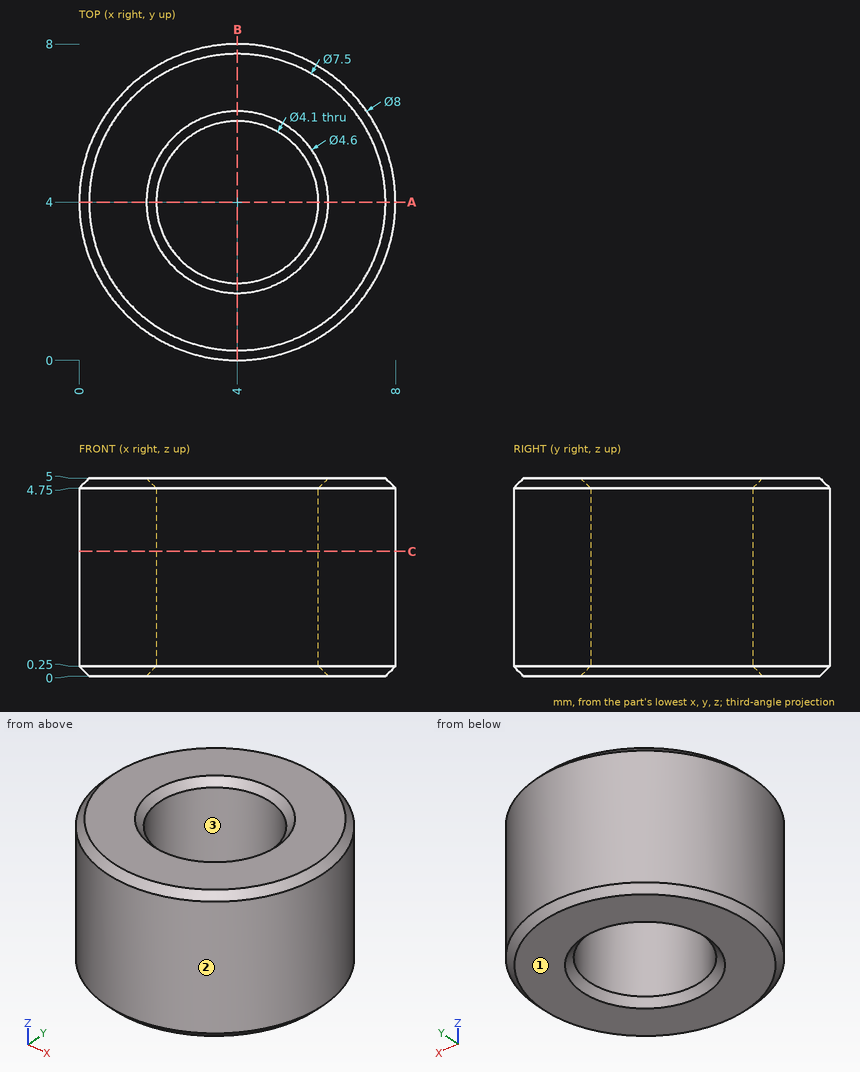
Can you work these out from the drawing? Everything is in mm from the part's minimum corner. Round coordinates to 2 decimals unless told otherwise and drop trailing zeros. Loops run counter-clockwise (first coordinate to the right, second up) from the corner with the lowest first, then second, coordinate; pieces in that order, holes last. Notation, with made-up numbers: (66.25, 16) - (112.25, 16) arc R15 cw to (112.25, 41) - close; hole circle Ø10 at (-31, -32). An arc over 180 degrees is marked (long way). One line per question, with ' | ' between items. Start each with the question number.
Q1. I want a section at A-A (y = 4). Write out the boundary of the cut face in (x, z), then the cut area to 4 significant figures.
Q2. We'd pull the mould along Y, two halves only. Please class the marked faces 1, 2 and 3: +Y half, -Y half, draft (parallel to the pull), parting line (faces both ways), or undercut.
Q3. Please list where these lines run through material, in increasing order: line 1 (Y direction, x = 4, z = 3.45); line 2 (X direction, y = 2.75, z = 3.45); line 3 (X direction, y = 3.5, z = 2.5). Write a range as [from, to].
Q4. I want a section at C-C (z = 3.15). Write out the boundary of the cut face in (x, y).
Q5. Will these pins go through, and if not, where does the flat tip stop? pin 1 (3 mm diameter, centred on x = 5.5, z = 2.5, fed in from +Y); pin 2 (2 mm diameter, centred on y = 6.5, z = 3, fed in from -X); pin 3 (1.5 mm diameter, centred on x = 2, z = 4, fed in from -Y).
Response values:
1) outline: (0, 0.25) - (0.25, 0) - (1.7, 0) - (1.95, 0.25) - (1.95, 4.75) - (1.7, 5) - (0.25, 5) - (0, 4.75) - close; (6.05, 0.25) - (6.3, 0) - (7.75, 0) - (8, 0.25) - (8, 4.75) - (7.75, 5) - (6.3, 5) - (6.05, 4.75) - close | area: 19.25 mm²
2) face 1: draft | face 2: parting line | face 3: undercut
3) line 1: y = [0, 1.95], [6.05, 8] | line 2: x = [0.2, 2.38], [5.62, 7.8] | line 3: x = [0.03, 2.01], [5.99, 7.97]
4) outline: circle Ø8 at (4, 4); hole circle Ø4.1 at (4, 4)
5) pin 1: stops at y = 8 | pin 2: stops at x = 0.29 | pin 3: stops at y = 0.2
